Could you check a few things on this model? Use its own coordinates, in mm. Face numbers are marked on the shaded views. A direction names the side the tool comes from. Round coordinates to 2 decimals unless told otherwise and drop trailing zeros. Write each loop counter-clockwise with the first axis right and the second up, starting at its lowest first coordinate (ties: lowest second). Pieces come first, ordered by that corner, then holes. Notation, with made-up numbers: (-20.5, -11) -> (24.5, -11) arc R22 ccw to (24.5, 1) -> close; hole circle Ø3 at (-36.5, -19.75). An arc over 180 degrees is marked (long way). Return JSON: item names as keys, results as strings.
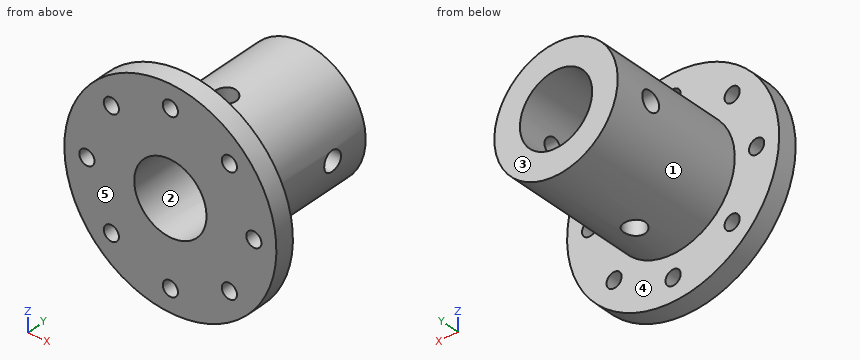
from build123d import *

# Parameters (mm, degrees)
SKETCH1_R               = 13.97
BOSS_EXTRUDE1_DEPTH     = 2.54
SKETCH2_R               = 8.128
BOSS_EXTRUDE2_DEPTH     = 18
SKETCH6_R               = 1
CUT_EXTRUDE2_DEPTH      = 29.499357888
SKETCH7_R               = 4.7625
CUT_EXTRUDE3_DEPTH      = 25.4
CUT_EXTRUDE6_DEPTH      = 24.13
CUT_EXTRUDE6_DEPTH_BACK = 24.13
SKETCH11_R              = 1.4
CUT_EXTRUDE7_DEPTH      = 29.49935796
CUT_EXTRUDE7_DEPTH_BACK = 29.49935796
SKETCH12_R              = 1.296623243


with BuildPart() as part:
    # Sketch1 → Boss-Extrude1 (new body)
    with BuildSketch(Plane(origin=(0, 0, 0), x_dir=(1, 0, 0), z_dir=(0, 1, 0))):
        with Locations(Location((0, 0, 0), (0, 0, 270))):
            Circle(SKETCH1_R)
    extrude(amount=BOSS_EXTRUDE1_DEPTH)

    # Sketch2 → Boss-Extrude2 (add)
    with BuildSketch(Plane(origin=(0, 2.54, 0), x_dir=(1, 0, 0), z_dir=(0, 1, 0))):
        with Locations(Location((0, 0, 0), (0, 0, 270))):
            Circle(SKETCH2_R)
    extrude(amount=BOSS_EXTRUDE2_DEPTH)

    # Sketch6 → Cut-Extrude2 (cut, through all)
    with BuildSketch(Plane(origin=(0, 0, 0), x_dir=(-1, 0, 0), z_dir=(0, -1, 0))):
        with Locations(Location((-11, 0, 0), (0, 0, 90))):
            Circle(SKETCH6_R)
        with Locations(Location((-7.778174593, 7.778174593, 0), (0, 0, 90))):
            Circle(SKETCH6_R)
        with Locations(Location((0, 11, 0), (0, 0, 90))):
            Circle(SKETCH6_R)
        with Locations(Location((7.778174593, 7.778174593, 0), (0, 0, 90))):
            Circle(SKETCH6_R)
        with Locations(Location((11, 0, 0), (0, 0, 90))):
            Circle(SKETCH6_R)
        with Locations(Location((7.778174593, -7.778174593, 0), (0, 0, 90))):
            Circle(SKETCH6_R)
        with Locations(Location((0, -11, 0), (0, 0, 90))):
            Circle(SKETCH6_R)
        with Locations(Location((-7.778174593, -7.778174593, 0), (0, 0, 90))):
            Circle(SKETCH6_R)
    extrude(amount=-CUT_EXTRUDE2_DEPTH, mode=Mode.SUBTRACT)

    # Sketch7 → Cut-Extrude3 (cut)
    with BuildSketch(Plane(origin=(0, 20.54, 0), x_dir=(1, 0, 0), z_dir=(0, 1, 0))):
        with Locations(Location((0, 0, 0), (0, 0, 270))):
            Circle(SKETCH7_R)
    extrude(amount=-CUT_EXTRUDE3_DEPTH, mode=Mode.SUBTRACT)

    # Sketch11 → Cut-Extrude6 (cut, two sides: drawn at the far end of the back side and taken through both)
    with BuildSketch(Plane.XY.offset(-CUT_EXTRUDE6_DEPTH_BACK)):
        with Locations(Location((0, 8.466000018, 0), (0, 0, 180))):
            Circle(SKETCH11_R)
    extrude(amount=CUT_EXTRUDE6_DEPTH + CUT_EXTRUDE6_DEPTH_BACK, mode=Mode.SUBTRACT)

    # Sketch12 → Cut-Extrude7 (cut, two sides: drawn at the far end of the back side and taken through both)
    with BuildSketch(Plane(origin=(0, 0, 0), x_dir=(0, 0, -1), z_dir=(1, 0, 0)).offset(-CUT_EXTRUDE7_DEPTH_BACK)):
        with Locations((0, 15.466)):
            Circle(SKETCH12_R)
    extrude(amount=CUT_EXTRUDE7_DEPTH + CUT_EXTRUDE7_DEPTH_BACK, mode=Mode.SUBTRACT)


solid = part.part
1) Thinking about a two-plate mould opening in Z: for the marked faces 1, 2 and 3, which applies, pulls with the +Z half, pulls with the -Z half, needs draft (parallel to the pull), parting line crosses it, or undercut?
Return value:
{"face 1": "parting line crosses it", "face 2": "undercut", "face 3": "needs draft"}
2) For the marked faces 4 and 5, which set-ups out of +Z, -Z, +X, -X, +Y, -Y let a thin tool reach every point of the face, with its end or its side?
Return value:
{"face 4": "+Y", "face 5": "+Z, -Z, +X, -X, -Y"}
3) I want a section at C-C, the plane z = 11. Please give me the cut outline in (x, y).
Return value:
{"outline": "(-8.61, 0) -> (-1, 0) -> (-1, 2.54) -> (-8.61, 2.54) -> close; (1, 0) -> (8.61, 0) -> (8.61, 2.54) -> (1, 2.54) -> close"}
4) I want a section at D-D, the plane y = 10.75. Please give me the cut outline in (x, z) (1 decimal).
Return value:
{"outline": "circle Ø16.3 at (0, 0); hole circle Ø9.5 at (0, 0)"}
5) If I drill on probe 1 along X at (y, z) = (2, 7.5); probe 2 along Y at (x, z) = (5.75, -6.5); probe 3 along Z at (x, y) = (0.5, 5.5), over which ranges is the centre line in solid material (lowest first)? Write a range as [from, to].
Return value:
{"probe 1": "[-11.79, -8.74], [-6.82, 6.82], [8.74, 11.79]", "probe 2": "[0, 2.54]", "probe 3": "[-8.11, -4.74], [4.74, 8.11]"}
6) Will these pins go through, and if not, where does the flat tip stop? pin 1 Ø8 at (x, y) = (9.5, 16) entering from +Z; pin 2 Ø3.5 at (y, z) = (15.466, 0) entering from -X; pin 3 Ø4 at (y, z) = (15, 5.5) entering from +X.
Return value:
{"pin 1": "z = 5.98", "pin 2": "x = -8.13", "pin 3": "x = 7.34"}
7) I want a section at B-B, the plane x = 0. Please give me the cut outline in (y, z), and give its area (3 significant figures).
Return value:
{"outline": "(0, -13.97) -> (2.54, -13.97) -> (2.54, -12) -> (0, -12) -> close; (0, -10) -> (2.54, -10) -> (2.54, -8.13) -> (7.07, -8.13) -> (7.07, -4.76) -> (0, -4.76) -> close; (0, 4.76) -> (7.07, 4.76) -> (7.07, 8.13) -> (2.54, 8.13) -> (2.54, 10) -> (0, 10) -> close; (0, 12) -> (2.54, 12) -> (2.54, 13.97) -> (0, 13.97) -> close; (9.87, -8.13) -> (20.54, -8.13) -> (20.54, -4.76) -> (9.87, -4.76) -> close; (9.87, 4.76) -> (20.54, 4.76) -> (20.54, 8.13) -> (9.87, 8.13) -> close", "area": "139 mm²"}
8) I want a section at A-A, the plane z = 0. Please give me the cut outline in (x, y).
Return value:
{"outline": "(-13.97, 0) -> (-12, 0) -> (-12, 2.54) -> (-13.97, 2.54) -> close; (-10, 0) -> (-4.76, 0) -> (-4.76, 14.17) -> (-8.13, 14.17) -> (-8.13, 2.54) -> (-10, 2.54) -> close; (-8.13, 16.76) -> (-4.76, 16.76) -> (-4.76, 20.54) -> (-8.13, 20.54) -> close; (4.76, 0) -> (10, 0) -> (10, 2.54) -> (8.13, 2.54) -> (8.13, 14.17) -> (4.76, 14.17) -> close; (4.76, 16.76) -> (8.13, 16.76) -> (8.13, 20.54) -> (4.76, 20.54) -> close; (12, 0) -> (13.97, 0) -> (13.97, 2.54) -> (12, 2.54) -> close"}
